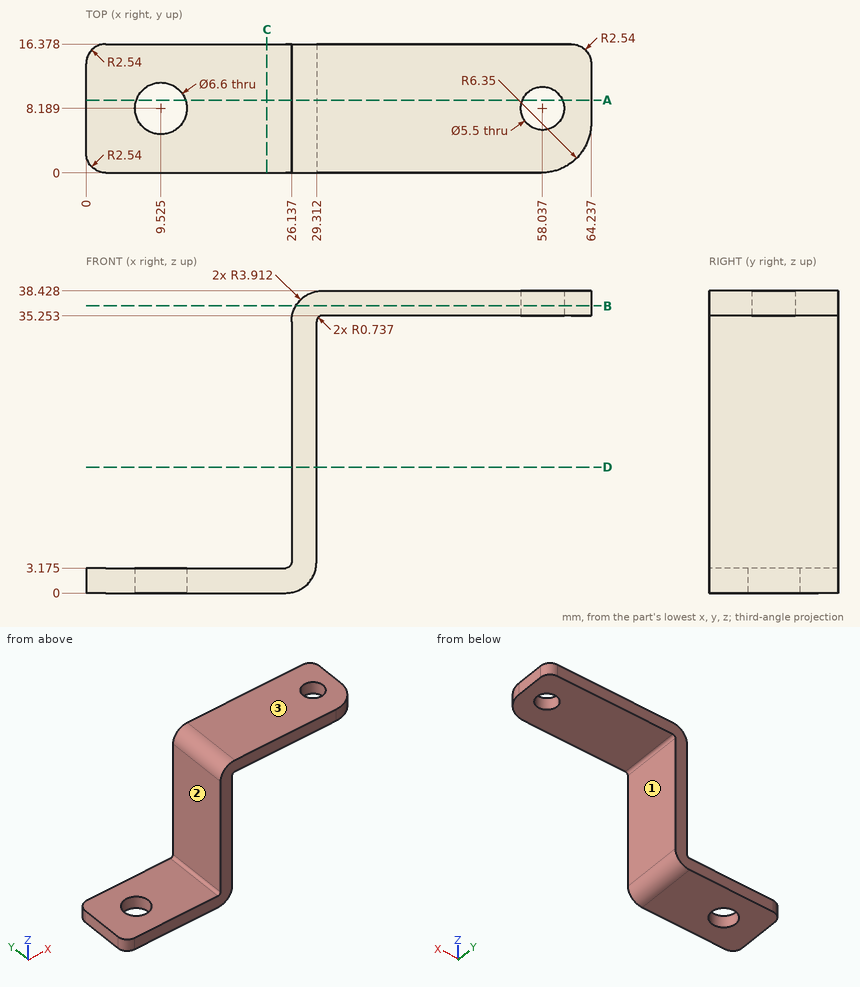
Here's the drawing with two shaded views (mm, measured from the low corner). I have some questions. A direction names the side the tool comes from. Coordinates: 2 decimals unless noted, no trailing zeros. Write each loop counter-clockwise with the first axis right and the second up, starting at its lowest first coordinate (ties: lowest second). Pieces come first, ordered by that corner, then holes. Notation, with made-up numbers: M 88.25,14.25 L 129.25,14.25 A21 ccw 129.25,22.25 Z; hole C 54.25,88.25 d9. An arc over 180 degrees is marked long. Answer as CSV lines item,"result".
Item 1: Imagine slicing it at B-B on z = 36.5. List the corners of the cut face in (x, y) for me, plus the area to 3 significant figures.
Geometry results:
outline,"M 26.68,0 L 57.89,0 A6.35 ccw 64.24,6.35 L 64.24,13.84 A2.54 ccw 61.7,16.38 L 26.68,16.38 Z; hole C 58.04,8.19 d5.5"
area,"581 mm2"
Item 2: On a 3-axis mill with a long thin cutter (end or side, diameter ignored), from which of +Z, -Z, +X, -X, +Y, -Y can I reach the whole of each face in a straight line? I mean the marked faces 1, 2 and 3. Say none if no direction works.
Geometry results:
face 1,"-Z, +X, +Y, -Y"
face 2,"+Z, -X, +Y, -Y"
face 3,"+Z, +X, -X, +Y, -Y"
Item 3: Imagine slicing it at D-D on z = 16. List the corners of the cut face in (x, y) for me, plus the area to 3 significant figures.
Geometry results:
outline,"M 26.14,0 L 29.31,0 L 29.31,16.38 L 26.14,16.38 Z"
area,"52.0 mm2"
Item 4: Imagine slicing it at A-A on y = 9.25. State how many separate pieces and enclosed holes the cut face has.
Geometry results:
separate pieces,"3"
enclosed holes,"0"
Item 5: Imagine slicing it at C-C on x = 23. List the corners of the cut face in (y, z) for me (1 decimal), plus the area to 3 significant figures.
Geometry results:
outline,"M 0,0 L 16.4,0 L 16.4,3.2 L 0,3.2 Z"
area,"52.0 mm2"
Item 6: I'm going to push flat-ended pins straight in: P1, Ø3, axis at y = 9, z = 21, coming from the +X side; P2, Ø1, axis at x = 48.5, y = 10, coming from the -Z side; P3, Ø8.5, axis at x = 9.525, y = 8.189, coming from the +Z side (3 decimals). Where does each tip first touch, or does it pass through?
Geometry results:
P1,"stops at x = 29.31"
P2,"stops at z = 35.25"
P3,"stops at z = 3.175"
Item 7: Please list where these lines run through material, in increasing order: line 1 along X through (y, z) = (6.5, 6.5); line 2 along Z through (x, y) = (50.5, 6.75); line 3 along Z through (x, y) = (15.5, 8.75) (1 decimal).
Geometry results:
line 1,"x = 26.14 to 29.31"
line 2,"z = 35.25 to 38.43"
line 3,"z = 0 to 3.2"
